Input: part model. Units: mm. Frame: model coordinates. A direction names the side the tool comes from. Round coordinates to 2 decimals unless told otherwise and drop trailing zeros. Loops run counter-clockwise (first coordinate to the right, second up) from the corner with the lowest first, then second, coordinate; pieces in that order, holes last. Notation, with made-up numbers: (45.25, -34) - (100.25, -34) arc R19 ccw to (100.25, -27) - close; hole circle Ø4 at (62, 12.25). An arc over 180 degrees is marked (long way). Use CSV: the item, a comma, the result in double quotes. Start each with the question number.
1. Material intervals for probe 1 along Z at (x, y) = (43.15, -51.2); probe 2 along Y at (x, z) = (53, -1.5); probe 3 along X at (y, z) = (-47.5, -17.5), sorted ascending. Write a range as from..to.
2. Cut plane A-A (x = 15). Return loops of the section in (y, z), and give its area (3 significant figures).
3. Cut plane D-D (x = 49). Return loops of the section in (y, z), and give its area (3 significant figures).
4. Pull-direction query (Z, two-part tool) for faces 1 (the cylindrical face through (56, -9, -12)), 2 (the flat face through (29, -5, -16)), 3 (the flat face through (29, -52, 0)); classes: +Z half, -Z half, draft (parallel to the pull), parting line (faces both ways), or undercut.
5. Access query for faces 4 (the cylindrical face through (44.34, -52.54, -6.37)), 5 (the flat face through (5, -28, -16)), 6 (the flat face through (29, -52, -31.5)). Directions: +Z, -Z, +X, -X, +Y, -Y. A direction counts if a zero-diameter tool reaches every point of the face in a straight line with its end or side. Return the directions, or none.
6. Cut plane C-C (y = -29). Return loops of the section in (x, z), and give its area (3 significant figures).
7. Cut plane B-B (z = -6.75). Return loops of the section in (x, y).
```python
from build123d import *

# Parameters (mm, degrees)
SKETCH_1_W          = 58.15
SKETCH_1_H          = 31.5
EXTRUDE_1_DEPTH     = 55
SKETCH_2_W          = 48.15
SKETCH_2_H          = 45
CUT_EXTRUDE_1_DEPTH = 31.5
SKETCH_4_R          = 1.25
CUT_EXTRUDE_2_DEPTH = 10
SKETCH_5_R          = 1.25
CUT_EXTRUDE_3_DEPTH = 10
SKETCH_6_R          = 1.25
CUT_EXTRUDE_4_DEPTH = 10


with BuildPart() as part:
    # 草图1 → 凸台-拉伸1 (new body)
    with BuildSketch(Plane(origin=(0, 0, 0), x_dir=(1, 0, 0), z_dir=(0, 1, 0))):
        with Locations((29.075, 15.75)):
            Rectangle(SKETCH_1_W, SKETCH_1_H)
    extrude(amount=-EXTRUDE_1_DEPTH)

    # 草图2 → 切除-拉伸1 (cut)
    with BuildSketch(Plane.XY):
        with Locations((29.075, -27.5)):
            Rectangle(SKETCH_2_W, SKETCH_2_H)
    extrude(amount=-CUT_EXTRUDE_1_DEPTH, mode=Mode.SUBTRACT)

    # 草图4 → 切除-拉伸2 (cut)
    with BuildSketch(Plane.XZ.offset(55)):
        with Locations((15, -6.75)):
            Circle(SKETCH_4_R)
        with Locations((15, -24.75)):
            Circle(SKETCH_4_R)
        with Locations((43.15, -6.75)):
            Circle(SKETCH_4_R)
        with Locations((43.15, -24.75)):
            Circle(SKETCH_4_R)
    extrude(amount=-CUT_EXTRUDE_2_DEPTH, mode=Mode.SUBTRACT)

    # 草图5 → 切除-拉伸3 (cut)
    with BuildSketch(Plane.ZY.offset(-53.15)):
        with Locations((-20.25, -10)):
            Circle(SKETCH_5_R)
        with Locations((-11.25, -10)):
            Circle(SKETCH_5_R)
    extrude(amount=-CUT_EXTRUDE_3_DEPTH, mode=Mode.SUBTRACT)

    # 草图6 → 切除-拉伸4 (cut)
    with BuildSketch(Plane(origin=(5, 0, 0), x_dir=(0, 0, -1), z_dir=(1, 0, 0))):
        with Locations((11.25, -10)):
            Circle(SKETCH_6_R)
        with Locations((20.25, -10)):
            Circle(SKETCH_6_R)
    extrude(amount=-CUT_EXTRUDE_4_DEPTH, mode=Mode.SUBTRACT)


solid = part.part
```
Established:
1,probe 1,"z = -31.5..-26, -23.5..-8, -5.5..0"
1,probe 2,"y = -55..-50, -5..0"
1,probe 3,"x = 0..5, 53.15..58.15"
2,outline,"(-55, -31.5) - (-50, -31.5) - (-50, -26) - (-55, -26) - close; (-55, -23.5) - (-50, -23.5) - (-50, -8) - (-55, -8) - close; (-55, -5.5) - (-50, -5.5) - (-50, 0) - (-55, 0) - close; (-5, -31.5) - (0, -31.5) - (0, 0) - (-5, 0) - close"
2,area,"290 mm2"
3,outline,"(-55, -31.5) - (-50, -31.5) - (-50, 0) - (-55, 0) - close; (-5, -31.5) - (0, -31.5) - (0, 0) - (-5, 0) - close"
3,area,"315 mm2"
4,face 1,"undercut"
4,face 2,"draft"
4,face 3,"+Z half"
5,face 4,"-Y"
5,face 5,"+Z, -Z"
5,face 6,"-Z, +X, -X, +Y, -Y"
6,outline,"(0, -31.5) - (5, -31.5) - (5, 0) - (0, 0) - close; (53.15, -31.5) - (58.15, -31.5) - (58.15, 0) - (53.15, 0) - close"
6,area,"315 mm2"
7,outline,"(0, -55) - (13.75, -55) - (13.75, -50) - (5, -50) - (5, -5) - (53.15, -5) - (53.15, -50) - (44.4, -50) - (44.4, -55) - (58.15, -55) - (58.15, 0) - (0, 0) - close; (16.25, -55) - (41.9, -55) - (41.9, -50) - (16.25, -50) - close"
